Verification items for the finished model (mm, model axes). Face numbers are marked on the shaded views. A direction names the side the tool comes from. Give positions to 0.01 mm unless a question says otherwise; leave off trailing zeros. Write each loop counter-clockwise with the first axis right and the second up, starting at its lowest first coordinate (ties: lowest second). Pieces come first, ordered by that corner, then holes. Notation, with made-up numbers: M 4,54 L 24,54 A20 cw 24,79 Z; hole C -26.75,15.25 d8. An arc over 180 degrees is marked long. Answer as a JSON object with one key per item and string values.
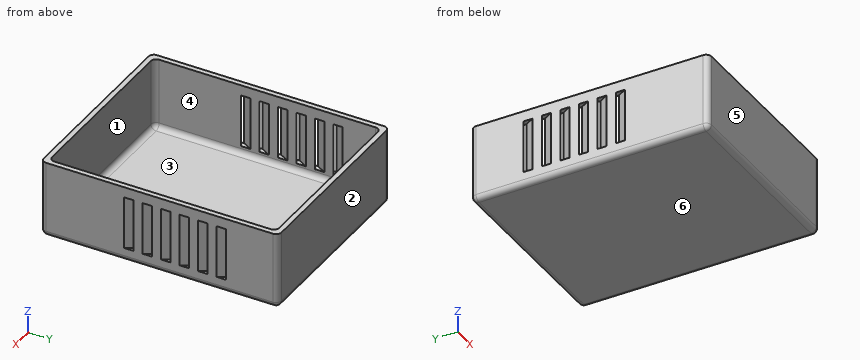
```python
from build123d import *

# Parameters (mm, degrees)
EXTRUDE007_DEPTH = 20
BOX003_W         = 70
BOX003_H         = 86
BOX003_DEPTH     = 39
FILLET001_R      = 2
BOX002_W         = 74
BOX002_H         = 90
BOX002_DEPTH     = 29
FILLET_R         = 2


with BuildPart() as ventsbottomcut:
    # Sketch007 → Extrude007 (new body)
    with BuildSketch(Plane.XY):
        Polygon((4, 77), (6, 76.999982), (-3.999992, 59.679487), (-5.999992, 59.679487), align=None)
        Polygon((-5.999992, 52.679487), (-3.999992, 52.679487), (6, 70), (4, 70), align=None)
        Polygon((-3.999992, 45.679487), (-5.999992, 45.679487), (4, 63), (6, 63), align=None)
        Polygon((4, 56), (6, 56), (-3.999992, 38.679487), (-5.999992, 38.679487), align=None)
        Polygon((4, 49), (6, 49), (-3.999992, 31.679487), (-5.999992, 31.679487), align=None)
        Polygon((4, 42), (6, 42), (-3.999992, 24.679487), (-5.999992, 24.679487), align=None)
        Polygon((70, 77), (68, 77), (78, 59.679492), (80, 59.679492), align=None)
        Polygon((68, 70), (70, 70), (80, 52.679492), (78, 52.679492), align=None)
        Polygon((68, 63), (70, 63), (80, 45.679492), (78, 45.679492), align=None)
        Polygon((68, 56), (70, 56), (80, 38.679492), (78, 38.679492), align=None)
        Polygon((68, 49), (70, 49), (80, 31.679492), (78, 31.679492), align=None)
        Polygon((68, 42), (70, 42), (80, 24.679492), (78, 24.679492), align=None)
    extrude(amount=EXTRUDE007_DEPTH)


with BuildPart() as ventsbottomcut_1:
    # Extrude007 placement: moved
    add(ventsbottomcut.part.moved(Location((0, 0, 5))))


with BuildPart() as bottomcut:
    # Box003 → Box003 (new body)
    with BuildSketch(Plane(origin=(2, 2, 2), x_dir=(1, 0, 0), z_dir=(0, 0, 1))):
        with Locations((35, 43)):
            Rectangle(BOX003_W, BOX003_H)
    extrude(amount=BOX003_DEPTH)

    # Fillet001
    fillet001_edges = [bottomcut.edges().sort_by_distance(p)[0] for p in [
        (2, 2, 21.5),
        (2, 88, 21.5),
        (2, 45, 2),
        (72, 2, 21.5),
        (72, 88, 21.5),
        (72, 45, 2),
        (37, 2, 2),
        (37, 88, 2),
    ]]
    fillet(fillet001_edges, radius=FILLET001_R)


with BuildPart() as bottom004done:
    # Box002 → Box002 (new body)
    with BuildSketch(Plane.XY):
        with Locations((37, 45)):
            Rectangle(BOX002_W, BOX002_H)
    extrude(amount=BOX002_DEPTH)

    # Fillet
    fillet_edges = [bottom004done.edges().sort_by_distance(p)[0] for p in [
        (0, 0, 14.5),
        (0, 90, 14.5),
        (0, 45, 0),
        (74, 0, 14.5),
        (74, 90, 14.5),
        (74, 45, 0),
        (37, 0, 0),
        (37, 90, 0),
    ]]
    fillet(fillet_edges, radius=FILLET_R)

    # Cut: cut bottomCut
    add(bottomcut.part, mode=Mode.SUBTRACT)

    # Cut002: cut ventsBottomCut
    add(ventsbottomcut_1.part, mode=Mode.SUBTRACT)


solid = bottom004done.part
```
1) Section check C-C on x = 44.5. Record the boundary of the cut face in (y, z), and give its area (3 significant figures).
Completed:
{"outline": "M 0,2 A2 ccw 2,0 L 88,0 A2 ccw 90,2 L 90,29 L 88,29 L 88,4 A2 cw 86,2 L 4,2 A2 cw 2,4 L 2,29 L 0,29 Z", "area": "288 mm2"}
2) Access from +Z, -Z, +X, -X, +Y, -Y to the whole of each face (thin tool, end or side, straight path). Record for the marked faces 1 and 2.
Completed:
{"face 1": "+Z", "face 2": "+Z, -Z, +X, -X, +Y"}
3) Section check B-B on y = 29.5. Record the boundary of the cut face in (x, z).
Completed:
{"outline": "M 0,2 A2 ccw 2,0 L 72,0 A2 ccw 74,2 L 74,29 L 72,29 L 72,4 A2 cw 70,2 L 4,2 A2 cw 2,4 L 2,29 L 0,29 Z"}
4) Thickness scan on L1, parallel to Y at x = 17, z = 10.75; L2, parallel to X at y = 31.5, z = 21; L3, parallel to Z at x = 61, y = 49.5. Record the ranges inside material, lowest first.
Completed:
{"L1": "y = 0 to 2, 88 to 90", "L2": "x = 0 to 2, 72 to 74", "L3": "z = 0 to 2"}
5) Go/stop test with flat-tipped pins: pin 1 (0.6 mm diameter, centred on x = 73.5, y = 36.5, fed in from -Z); pin 2 (1 mm diameter, centred on x = 73, y = 42.5, fed in from -Z); pin 3 (1.6 mm diameter, centred on x = 1, y = 71.5, fed in from -Z). Record where each tip stops, or that it passes through.
Completed:
{"pin 1": "stops at z = 0.4", "pin 2": "stops at z = 0.06", "pin 3": "stops at z = 0.01"}
6) Section check D-D on z = 19. Count the separate pieces of the cut face and the enclosed holes in it, and give its area (3 significant figures).
Completed:
{"separate pieces": "12", "enclosed holes": "0", "area": "557 mm2"}
7) Section check A-A on z = 26. Record the boundary of the cut face in (x, y), and give its area (3 significant figures).
Completed:
{"outline": "M 0,2 A2 ccw 2,0 L 72,0 A2 ccw 74,2 L 74,88 A2 ccw 72,90 L 2,90 A2 ccw 0,88 Z; hole M 2,4 A2 ccw 4,2 L 70,2 A2 ccw 72,4 L 72,86 A2 ccw 70,88 L 4,88 A2 ccw 2,86 Z", "area": "640 mm2"}
8) Release check for a two-part mould opening along Y. For the marked faces 3, 4, 5 and 6 record: pulls with the +Y half, pulls with the -Y half, needs draft (parallel to the pull), parting line crosses it, or undercut.
Completed:
{"face 3": "undercut", "face 4": "undercut", "face 5": "pulls with the -Y half", "face 6": "needs draft"}
